```python
from build123d import *

# Parameters (mm, degrees)
SKETCH2_R           = 3
CUT_EXTRUDE3_DEPTH  = 100
BOSS_EXTRUDE1_REACH = 129.709
SKETCH3_R           = 5
SKETCH3_R_2         = 3


with BuildPart() as part:
    # Sketch1 → Revolve1 (revolve)
    with BuildSketch(Plane.XY, mode=Mode.PRIVATE) as revolve1_sk:
        with BuildLine():
            Line((3.8, 0), (3.8, -15))
            Line((3.8, -15), (1.5, -15))
            Line((1.5, -15), (1.5, 0))
            add(Edge.make_bspline(
                [(81.5, 40), (1.5, 40), (1.5, 0)],
                knots=[4.71238898, 4.71238898, 4.71238898, 6.283185307, 6.283185307, 6.283185307], degree=2, weights=[1, 0.707106781, 1]))
            Line((81.5, 40), (81.5, 36.5))
            add(Edge.make_bspline(
                [(3.8, 0), (3.8, 6.33566197), (17.718114252, 21.385939358), (45.345693135, 33.248700069), (66.206013583, 36.5), (81.5, 36.5)],
                knots=[0, 0, 0, 0, 0.319283378, 0.419283378, 1, 1, 1, 1], degree=3))
        make_face()
    revolve(revolve1_sk.sketch.rotate(Axis((0, 59.506196768, 0), (0, -1, 0)), 90), axis=Axis((0, 59.506196768, 0), (0, -1, 0)))

    # Sketch2 → Cut-Extrude3 (cut)
    with BuildSketch(Plane(origin=(0, 0, 0), x_dir=(1, 0, 0), z_dir=(0, 1, 0))):
        with Locations(Location((-40, 40, 0), (0, 0, 90))):
            Circle(SKETCH2_R)
        with Locations(Location((40, 40, 0), (0, 0, 90))):
            Circle(SKETCH2_R)
        with Locations(Location((40, -40, 0), (0, 0, 90))):
            Circle(SKETCH2_R)
        with Locations(Location((-40, -40, 0), (0, 0, 90))):
            Circle(SKETCH2_R)
    extrude(amount=CUT_EXTRUDE3_DEPTH, mode=Mode.SUBTRACT)

    # Sketch3 → Boss-Extrude1 (add, up to next)
    with BuildSketch(Plane(origin=(0, 40, 0), x_dir=(1, 0, 0), z_dir=(0, 1, 0)), mode=Mode.PRIVATE) as boss_extrude1_sk1:
        with Locations(Location((40, 40, 0), (0, 0, 270))):
            Circle(SKETCH3_R)
        with Locations(Location((40, 40, 0), (0, 0, 90))):
            Circle(SKETCH3_R_2, mode=Mode.SUBTRACT)
    boss_extrude1_tool1 = extrude(boss_extrude1_sk1.sketch, amount=-BOSS_EXTRUDE1_REACH, mode=Mode.PRIVATE) - part.part
    # Sketch3 → Boss-Extrude1 (add, up to next)
    with BuildSketch(Plane(origin=(0, 40, 0), x_dir=(1, 0, 0), z_dir=(0, 1, 0)), mode=Mode.PRIVATE) as boss_extrude1_sk2:
        with Locations(Location((-40, 40, 0), (0, 0, 270))):
            Circle(SKETCH3_R)
        with Locations(Location((-40, 40, 0), (0, 0, 90))):
            Circle(SKETCH3_R_2, mode=Mode.SUBTRACT)
    boss_extrude1_tool2 = extrude(boss_extrude1_sk2.sketch, amount=-BOSS_EXTRUDE1_REACH, mode=Mode.PRIVATE) - part.part
    # Sketch3 → Boss-Extrude1 (add, up to next)
    with BuildSketch(Plane(origin=(0, 40, 0), x_dir=(1, 0, 0), z_dir=(0, 1, 0)), mode=Mode.PRIVATE) as boss_extrude1_sk3:
        with Locations(Location((-40, -40, 0), (0, 0, 270))):
            Circle(SKETCH3_R)
        with Locations(Location((-40, -40, 0), (0, 0, 90))):
            Circle(SKETCH3_R_2, mode=Mode.SUBTRACT)
    boss_extrude1_tool3 = extrude(boss_extrude1_sk3.sketch, amount=-BOSS_EXTRUDE1_REACH, mode=Mode.PRIVATE) - part.part
    # Sketch3 → Boss-Extrude1 (add, up to next)
    with BuildSketch(Plane(origin=(0, 40, 0), x_dir=(1, 0, 0), z_dir=(0, 1, 0)), mode=Mode.PRIVATE) as boss_extrude1_sk4:
        with Locations(Location((40, -40, 0), (0, 0, 270))):
            Circle(SKETCH3_R)
        with Locations(Location((40, -40, 0), (0, 0, 90))):
            Circle(SKETCH3_R_2, mode=Mode.SUBTRACT)
    boss_extrude1_tool4 = extrude(boss_extrude1_sk4.sketch, amount=-BOSS_EXTRUDE1_REACH, mode=Mode.PRIVATE) - part.part
    add(boss_extrude1_tool1.solids().sort_by_distance((40, 40, -44.858579))[0])
    add(boss_extrude1_tool2.solids().sort_by_distance((-40, 40, -44.858579))[0])
    add(boss_extrude1_tool3.solids().sort_by_distance((-40, 40, 35.141421))[0])
    add(boss_extrude1_tool4.solids().sort_by_distance((40, 40, 35.141421))[0])


solid = part.part
```
For this review, take the finished solid that the model builds, in its own axes (mm). A direction names the side the tool comes from. Coordinates: 2 decimals unless noted, no trailing zeros. Use one line per item in the form item = value. Start each with the question number.
1) To check wall thickness, follow probe 1 along Z at (x, y) = (40, 38); probe 2 along Y at (x, z) = (-52, 13.5); probe 3 along X at (y, z) = (34, 40). State the ranges of each line that lie inside material, in increasing order. Write a range as from..to.
2) For pin 1 (5 mm diameter, centred on x = -40, z = -40, fed in from +Y) (3 decimals); pin 2 (8 mm diameter, centred on x = -45.5, z = -58.5, fed in from -Y); pin 3 (4 mm diameter, centred on x = -10, z = -59.5, fed in from -Y); pin 4 (10 mm diameter, centred on y = -1.5, z = -1, fed in from -X), all flat-tipped, find the tip position at first contact; note any pin that passes through.
3) Take a section at A-A (x = 40). State how many separate pieces and enclosed holes the cut face has, plus the area to 3 significant figures.
4) For faces 5 (the face through (-43.3, 40, -40.1)), 6 (the face through (-1.141, -7.605, 3.625)), list the 3-axis set-ups (+Z, -Z, +X, -X, +Y, -Y) from which the entire face can be reached by the end or side of a thin tool; tool diameter is ignored.
5) Draft analysis for pull direction Z (two halves, no side actions). For faces 1 (the face through (-37, 39, 36)), 2 (the face through (-43.3, 40, 39.9)), 3 (the face through (31.215, 38.226, 75.285)), 4 (the face through (35.564, 38.89, -37.693)), state which applies: released by +Z, released by -Z, zero draft, split by the parting line, or undercut.
From the geometry:
q1.probe_1 = -71.01..-43, -37..-35, 35..37, 43..71.01
q1.probe_2 = 33.68..37.51
q1.probe_3 = -37..37
q2.pin_1 = through
q2.pin_2 = 36.01
q2.pin_3 = 34.53
q2.pin_4 = -4.58
q3.separate_pieces = 3
q3.enclosed_holes = 0
q3.area = 511 mm2
q4.face_5 = +Z, -Z, +X, -X, +Y
q4.face_6 = -Y
q5.face_1 = undercut
q5.face_2 = zero draft
q5.face_3 = split by the parting line
q5.face_4 = undercut
